Check sheet for the modelled part. Datum: model origin and axes. Units: mm. A direction names the side the tool comes from. Give positions to 0.01 mm unless a question says otherwise; leave off trailing zeros. Order: outer loops, then holes, each group sorted by start corner. A loop starts at its lowest first (then second) coordinate and runs counter-clockwise, first axis right, second up.
```python
from build123d import *

# Parameters (mm, degrees)
SKETCH2_R           = 1.6
BOSS_EXTRUDE1_DEPTH = 15
SKETCH3_R           = 1.6
BOSS_EXTRUDE2_DEPTH = 5
SKETCH4_R           = 2.8
CUT_EXTRUDE1_DEPTH  = 3
FILLET3_R           = 2
FILLET4_R           = 0.5


with BuildPart() as part:
    # Sketch2 → Boss-Extrude1 (new body)
    # profile 1 of 5: a face of its own
    with BuildSketch(Plane(origin=(0, 5.1, 0), x_dir=(1, 0, 0), z_dir=(0, 1, 0))):
        with BuildLine():
            Line((-27.3, -29.5), (-27.3, -25.1))
            Line((-27.3, -25.1), (-30.1, -25.1))
            ThreePointArc((-30.1, -25.1), (-32.221320344, -24.221320344), (-33.1, -22.1))
            Line((-33.1, -22.1), (-33.1, -18.8))
            Line((-33.1, -18.8), (-33.1, 18.5))
            Line((-33.1, 18.5), (-33.1, 22.1))
            ThreePointArc((-33.1, 22.1), (-32.221320344, 24.221320344), (-30.1, 25.1))
            Line((-30.1, 25.1), (-26.5, 25.1))
            Line((-26.5, 25.1), (26.5, 25.1))
            Line((26.5, 25.1), (30.1, 25.1))
            ThreePointArc((30.1, 25.1), (32.221320344, 24.221320344), (33.1, 22.1))
            Line((33.1, 22.1), (33.1, 18.5))
            Line((33.1, 18.5), (33.1, -18.8))
            Line((33.1, -18.8), (33.1, -22.1))
            ThreePointArc((33.1, -22.1), (32.221320344, -24.221320344), (30.1, -25.1))
            Line((30.1, -25.1), (27.3, -25.1))
            Line((27.3, -25.1), (27.3, -29.5))
            Line((27.3, -29.5), (31.5, -29.5))
            ThreePointArc((31.5, -29.5), (35.742640687, -27.742640687), (37.5, -23.5))
            Line((37.5, -23.5), (37.5, 23.5))
            ThreePointArc((37.5, 23.5), (35.742640687, 27.742640687), (31.5, 29.5))
            Line((31.5, 29.5), (-31.5, 29.5))
            ThreePointArc((-31.5, 29.5), (-35.742640687, 27.742640687), (-37.5, 23.5))
            Line((-37.5, 23.5), (-37.5, -23.5))
            ThreePointArc((-37.5, -23.5), (-35.742640687, -27.742640687), (-31.5, -29.5))
            Line((-31.5, -29.5), (-27.3, -29.5))
        make_face()
    # profile 2 of 5: a face of its own
    with BuildSketch(Plane(origin=(0, 5.1, 0), x_dir=(1, 0, 0), z_dir=(0, 1, 0))):
        with BuildLine():
            Line((-33.1, 22.1), (-33.1, 18.5))
            ThreePointArc((-33.1, 18.5), (-32.953553391, 18.853553391), (-32.6, 19))
            Line((-32.6, 19), (-30, 19))
            ThreePointArc((-30, 19), (-27.878679656, 19.878679656), (-27, 22))
            Line((-27, 22), (-27, 24.6))
            ThreePointArc((-27, 24.6), (-26.853553391, 24.953553391), (-26.5, 25.1))
            Line((-26.5, 25.1), (-30.1, 25.1))
            ThreePointArc((-30.1, 25.1), (-32.221320344, 24.221320344), (-33.1, 22.1))
        make_face()
        with Locations(Location((-30, 22, 0), (0, 0, 270))):
            Circle(SKETCH2_R, mode=Mode.SUBTRACT)
    # profile 3 of 5: a face of its own
    with BuildSketch(Plane(origin=(0, 5.1, 0), x_dir=(1, 0, 0), z_dir=(0, 1, 0))):
        with BuildLine():
            ThreePointArc((32.6, 19), (32.953553391, 18.853553391), (33.1, 18.5))
            Line((33.1, 18.5), (33.1, 22.1))
            ThreePointArc((33.1, 22.1), (32.221320344, 24.221320344), (30.1, 25.1))
            Line((30.1, 25.1), (26.5, 25.1))
            ThreePointArc((26.5, 25.1), (26.853553391, 24.953553391), (27, 24.6))
            Line((27, 24.6), (27, 22))
            ThreePointArc((27, 22), (27.878679656, 19.878679656), (30, 19))
            Line((30, 19), (32.6, 19))
        make_face()
        with Locations(Location((30, 22, 0), (0, 0, 270))):
            Circle(SKETCH2_R, mode=Mode.SUBTRACT)
    # profile 4 of 5: a face of its own
    with BuildSketch(Plane(origin=(0, 5.1, 0), x_dir=(1, 0, 0), z_dir=(0, 1, 0))):
        with BuildLine():
            Line((27.3, -22), (27.3, -25.1))
            Line((27.3, -25.1), (30.1, -25.1))
            ThreePointArc((30.1, -25.1), (32.221320344, -24.221320344), (33.1, -22.1))
            Line((33.1, -22.1), (33.1, -18.8))
            ThreePointArc((33.1, -18.8), (32.953553391, -19.153553391), (32.6, -19.3))
            Line((32.6, -19.3), (30, -19.3))
            ThreePointArc((30, -19.3), (28.090811691, -20.090811691), (27.3, -22))
        make_face()
        with Locations(Location((30, -22, 0), (0, 0, 270))):
            Circle(SKETCH2_R, mode=Mode.SUBTRACT)
    # profile 5 of 5: a face of its own
    with BuildSketch(Plane(origin=(0, 5.1, 0), x_dir=(1, 0, 0), z_dir=(0, 1, 0))):
        with BuildLine():
            Line((-27.3, -25.1), (-27.3, -22))
            ThreePointArc((-27.3, -22), (-28.090811691, -20.090811691), (-30, -19.3))
            Line((-30, -19.3), (-32.6, -19.3))
            ThreePointArc((-32.6, -19.3), (-32.953553391, -19.153553391), (-33.1, -18.8))
            Line((-33.1, -18.8), (-33.1, -22.1))
            ThreePointArc((-33.1, -22.1), (-32.221320344, -24.221320344), (-30.1, -25.1))
            Line((-30.1, -25.1), (-27.3, -25.1))
        make_face()
        with Locations(Location((-30, -22, 0), (0, 0, 270))):
            Circle(SKETCH2_R, mode=Mode.SUBTRACT)
    extrude(amount=BOSS_EXTRUDE1_DEPTH)

    # Sketch3 → Boss-Extrude2 (add)
    # profile 1 of 2: a face of its own
    with BuildSketch(Plane(origin=(0, 20.1, 0), x_dir=(1, 0, 0), z_dir=(0, 1, 0))):
        with BuildLine():
            ThreePointArc((-30, -19.3), (-28.090811691, -20.090811691), (-27.3, -22))
            Line((-27.3, -22), (-27.3, -19.2))
            Line((-27.3, -19.2), (27.3, -19.2))
            Line((27.3, -19.2), (27.3, -22))
            ThreePointArc((27.3, -22), (28.090811691, -20.090811691), (30, -19.3))
            Line((30, -19.3), (32.6, -19.3))
            ThreePointArc((32.6, -19.3), (32.953553391, -19.153553391), (33.1, -18.8))
            Line((33.1, -18.8), (33.1, 18.5))
            ThreePointArc((33.1, 18.5), (32.953553391, 18.853553391), (32.6, 19))
            Line((32.6, 19), (30, 19))
            ThreePointArc((30, 19), (27.878679656, 19.878679656), (27, 22))
            Line((27, 22), (27, 24.6))
            ThreePointArc((27, 24.6), (26.853553391, 24.953553391), (26.5, 25.1))
            Line((26.5, 25.1), (-26.5, 25.1))
            ThreePointArc((-26.5, 25.1), (-26.853553391, 24.953553391), (-27, 24.6))
            Line((-27, 24.6), (-27, 22))
            ThreePointArc((-27, 22), (-27.878679656, 19.878679656), (-30, 19))
            Line((-30, 19), (-32.6, 19))
            ThreePointArc((-32.6, 19), (-32.953553391, 18.853553391), (-33.1, 18.5))
            Line((-33.1, 18.5), (-33.1, -18.8))
            ThreePointArc((-33.1, -18.8), (-32.953553391, -19.153553391), (-32.6, -19.3))
            Line((-32.6, -19.3), (-30, -19.3))
        make_face()
    # profile 2 of 2: a face of its own
    with BuildSketch(Plane(origin=(0, 20.1, 0), x_dir=(1, 0, 0), z_dir=(0, 1, 0))):
        with BuildLine():
            Line((32.6, -19.3), (30, -19.3))
            ThreePointArc((30, -19.3), (28.090811691, -20.090811691), (27.3, -22))
            Line((27.3, -22), (27.3, -29.5))
            Line((27.3, -29.5), (31.5, -29.5))
            ThreePointArc((31.5, -29.5), (35.742640687, -27.742640687), (37.5, -23.5))
            Line((37.5, -23.5), (37.5, 23.5))
            ThreePointArc((37.5, 23.5), (35.742640687, 27.742640687), (31.5, 29.5))
            Line((31.5, 29.5), (-31.5, 29.5))
            ThreePointArc((-31.5, 29.5), (-35.742640687, 27.742640687), (-37.5, 23.5))
            Line((-37.5, 23.5), (-37.5, -23.5))
            ThreePointArc((-37.5, -23.5), (-35.742640687, -27.742640687), (-31.5, -29.5))
            Line((-31.5, -29.5), (-27.3, -29.5))
            Line((-27.3, -29.5), (-27.3, -22))
            ThreePointArc((-27.3, -22), (-28.090811691, -20.090811691), (-30, -19.3))
            Line((-30, -19.3), (-32.6, -19.3))
            ThreePointArc((-32.6, -19.3), (-32.953553391, -19.153553391), (-33.1, -18.8))
            Line((-33.1, -18.8), (-33.1, 18.5))
            ThreePointArc((-33.1, 18.5), (-32.953553391, 18.853553391), (-32.6, 19))
            Line((-32.6, 19), (-30, 19))
            ThreePointArc((-30, 19), (-27.878679656, 19.878679656), (-27, 22))
            Line((-27, 22), (-27, 24.6))
            ThreePointArc((-27, 24.6), (-26.853553391, 24.953553391), (-26.5, 25.1))
            Line((-26.5, 25.1), (26.5, 25.1))
            ThreePointArc((26.5, 25.1), (26.853553391, 24.953553391), (27, 24.6))
            Line((27, 24.6), (27, 22))
            ThreePointArc((27, 22), (27.878679656, 19.878679656), (30, 19))
            Line((30, 19), (32.6, 19))
            ThreePointArc((32.6, 19), (32.953553391, 18.853553391), (33.1, 18.5))
            Line((33.1, 18.5), (33.1, -18.8))
            ThreePointArc((33.1, -18.8), (32.953553391, -19.153553391), (32.6, -19.3))
        make_face()
        with Locations(Location((30, -22, 0), (0, 0, 270))):
            Circle(SKETCH3_R, mode=Mode.SUBTRACT)
        with Locations(Location((-30, 22, 0), (0, 0, 270))):
            Circle(SKETCH3_R, mode=Mode.SUBTRACT)
        with Locations(Location((-30, -22, 0), (0, 0, 270))):
            Circle(SKETCH3_R, mode=Mode.SUBTRACT)
        with Locations(Location((30, 22, 0), (0, 0, 270))):
            Circle(SKETCH3_R, mode=Mode.SUBTRACT)
    extrude(amount=BOSS_EXTRUDE2_DEPTH)

    # Sketch4 → Cut-Extrude1 (cut)
    with BuildSketch(Plane(origin=(0, 25.1, 0), x_dir=(1, 0, 0), z_dir=(0, 1, 0))):
        with Locations(Location((-30, 22, 0), (0, 0, 270))):
            Circle(SKETCH4_R)
        with Locations(Location((30, 22, 0), (0, 0, 90))):
            Circle(SKETCH4_R)
        with BuildLine():
            Line((-30, -19.2), (-27.3, -19.2))
            Line((-27.3, -19.2), (-27.3, -24.8))
            Line((-27.3, -24.8), (-30, -24.8))
            ThreePointArc((-30, -24.8), (-32.8, -22), (-30, -19.2))
        make_face()
        with BuildLine():
            Line((27.3, -19.2), (27.3, -24.8))
            Line((27.3, -24.8), (30, -24.8))
            ThreePointArc((30, -24.8), (32.8, -22), (30, -19.2))
            Line((30, -19.2), (27.3, -19.2))
        make_face()
    extrude(amount=-CUT_EXTRUDE1_DEPTH, mode=Mode.SUBTRACT)

    # Fillet3
    fillet3_edges = [part.edges().sort_by_distance(p)[0] for p in [
        (29.4, 25.1, 29.5),
        (35.742640687, 25.1, 27.742640687),
        (37.5, 25.1, 0),
        (35.742640687, 25.1, -27.742640687),
        (0, 25.1, -29.5),
        (-35.742640687, 25.1, -27.742640687),
        (-37.5, 25.1, 0),
        (-35.742640687, 25.1, 27.742640687),
        (-29.4, 25.1, 29.5),
    ]]
    fillet(fillet3_edges, radius=FILLET3_R)

    # Fillet4
    fillet4_edges = [part.edges().sort_by_distance(p)[0] for p in [
        (27.3, 25.1, 26.15),
        (-27.3, 25.1, 26.15),
        (27.3, 14.1, 29.5),
        (27.3, 24.514213562, 28.914213562),
        (-27.3, 14.1, 29.5),
        (-27.3, 24.514213562, 28.914213562),
    ]]
    fillet(fillet4_edges, radius=FILLET4_R)


solid = part.part
```
(1) Tool access check on faces 1 (the face through (-27, 12, -23)), 2 (the face through (32, 22.1, -22)), 3 (the face through (27.3, 15, 25)), 4 (the face through (-33.1, 12, 0)). Record the directions out of +Z, -Z, +X, -X, +Y, -Y that give a thin tool (end or side, any length) a straight path to the whole face; none if there is none.
(2) Thickness scan on L1, parallel to X at y = 17.5, z = -22; L2, parallel to X at y = 9.5, z = 22; L3, parallel to Z at x = -30, y = 13.25. Record the ranges inside material, lowest first.
(3) Sectioned sample at A-A (z = -17). Enter the section's corners in (x, y), plus the area to 3 significant figures.
(4) Sectioned sample at B-B (x = 0). Enter the section's corners in (y, z), plus the area to 3 significant figures.
(5) Go/stop test with flat-tipped pins: P1, Ø4, axis at x = 30, z = 22, coming from the +Y side; P2, Ø8, axis at x = -10.5, y = 10, coming from the +Z side; P3, Ø0.8, axis at x = -29, y = 23.5, coming from the -Z side; P4, Ø3, axis at x = -30, z = 22, coming from the +Y side. Record where each tip stops, or that it passes through.
(6) Release check for a two-part mould opening along Z. For faces 5 (the face through (0, 14, -29.5)), 6 (the face through (-29, 24, 24.8)), 7 (the face through (-27.3, 15, 25)), 8 (the face through (30, 14, 29.5)) record: released by +Z, released by -Z, zero draft, split by the parting line, or undercut.
(7) Sectioned sample at C-C (y = 11.75). Count the separate pieces of the cut face and the enclosed holes in it, plus the area to 3 significant figures.
Values follow:
1. face 1: +Z, -Y
1. face 2: +Y
1. face 3: +Z, +Y, -Y
1. face 4: -Y
2. L1: x = -37.5 to -31.6, -28.4 to -27, 27 to 28.4, 31.6 to 37.5
2. L2: x = -37.5 to -31.6, -28.4 to -27.3, 27.3 to 28.4, 31.6 to 37.5
2. L3: z = -29.5 to -23.6, -20.4 to -19, 19.3 to 20.4, 23.6 to 29.5
3. outline: (-37.5, 5.1) - (-33.1, 5.1) - (-33.1, 20.1) - (33.1, 20.1) - (33.1, 5.1) - (37.5, 5.1) - (37.5, 23.1) arc R2 ccw to (35.5, 25.1) - (-35.5, 25.1) arc R2 ccw to (-37.5, 23.1) - close
3. area: 505 mm2
4. outline: (5.1, -29.5) - (23.1, -29.5) arc R2 ccw to (25.1, -27.5) - (25.1, 19.2) - (20.1, 19.2) - (20.1, -25.1) - (5.1, -25.1) - close
4. area: 309 mm2
5. P1: stops at y = 22.1
5. P2: stops at z = -25.1
5. P3: stops at z = -29.5
5. P4: passes through
6. face 5: released by -Z
6. face 6: undercut
6. face 7: zero draft
6. face 8: released by +Z
7. separate pieces: 1
7. enclosed holes: 4
7. area: 933 mm2
